Can you work these out from the drawing? Everything is in mm from the part's minimum corner. A direction names the side the tool comes from. Give positions to 0.01 mm unless a question says otherwise; leave off trailing zeros. Write each loop counter-clockwise with the first axis right and the second up, starting at its lowest first coordinate (ties: lowest second). Pieces come first, ordered by that corner, then holes. Notation, with made-up numbers: (-12.75, 15.25) - (19.25, 15.25) arc R14 cw to (19.25, 33.25) - close; hole circle Ø10 at (-32, 82). An arc over 180 degrees is marked (long way). Use a Markdown table: item, result.
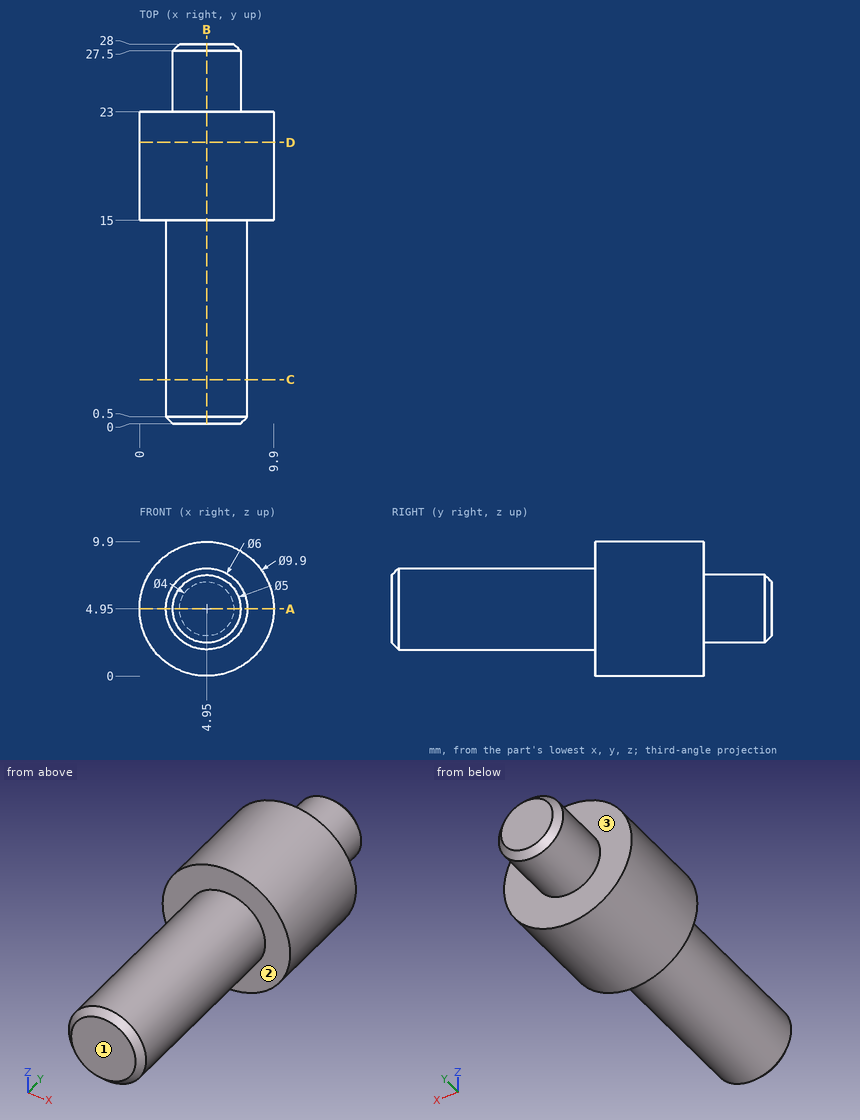
Item 1: I need wall thicknesses on line 1 along Y through (x, z) = (2, 1.75); line 2 along X through (y, z) = (13.25, 5); line 3 along Z through (x, y) = (7, 24.5). Which ranges of each line are inside material? Lowest first, please. Write a range as [from, to].
Values:
| item | result |
|---|---|
| line 1 | y = [15, 23] |
| line 2 | x = [1.95, 7.95] |
| line 3 | z = [3.52, 6.38] |
Item 2: If we section it at C-C, the plane y = 3.25: Write out the boundary of the cut face in (x, z), plus the area to 3 significant figures.
Values:
| item | result |
|---|---|
| outline | circle Ø6 at (4.95, 4.95) |
| area | 28.3 mm2 |
Item 3: If we section it at B-B, the plane x = 4.95: Write out the boundary of the cut face in (y, z), plus the area to 3 significant figures.
Values:
| item | result |
|---|---|
| outline | (0, 2.45) - (0.5, 1.95) - (15, 1.95) - (15, 0) - (23, 0) - (23, 2.45) - (27.5, 2.45) - (28, 2.95) - (28, 6.95) - (27.5, 7.45) - (23, 7.45) - (23, 9.9) - (15, 9.9) - (15, 7.95) - (0.5, 7.95) - (0, 7.45) - close |
| area | 194 mm2 |
Item 4: For the marked faces 1, 2 and 3, which set-ups out of +Z, -Z, +X, -X, +Y, -Y let a thin tool reach every point of the face, with its end or its side?
Values:
| item | result |
|---|---|
| face 1 | +Z, -Z, +X, -X, -Y |
| face 2 | -Y |
| face 3 | +Y |
Item 5: If we section it at D-D, the plane y = 20.75: Write out the boundary of the cut face in (x, z).
Values:
| item | result |
|---|---|
| outline | circle Ø9.9 at (4.95, 4.95) |
Item 6: Will these pins go through, and if not, where does the flat tip stop? pin 1 Ø1.5 at (x, y) = (2, 16.5) entering from -Z; pin 2 Ø5 at (x, z) = (5, 7.5) entering from +Y; pin 3 Ø2 at (y, z) = (3, 5) entering from -X; pin 4 Ø5 at (x, y) = (5.5, 9) entering from -Z.
Values:
| item | result |
|---|---|
| pin 1 | stops at z = 0.52 |
| pin 2 | stops at y = 28 |
| pin 3 | stops at x = 1.95 |
| pin 4 | stops at z = 1.95 |
Item 7: If we section it at A-A, the plane z = 4.95: Write out the boundary of the cut face in (x, y), plus the area to 3 significant figures.
Values:
| item | result |
|---|---|
| outline | (0, 15) - (1.95, 15) - (1.95, 0.5) - (2.45, 0) - (7.45, 0) - (7.95, 0.5) - (7.95, 15) - (9.9, 15) - (9.9, 23) - (7.45, 23) - (7.45, 27.5) - (6.95, 28) - (2.95, 28) - (2.45, 27.5) - (2.45, 23) - (0, 23) - close |
| area | 194 mm2 |
